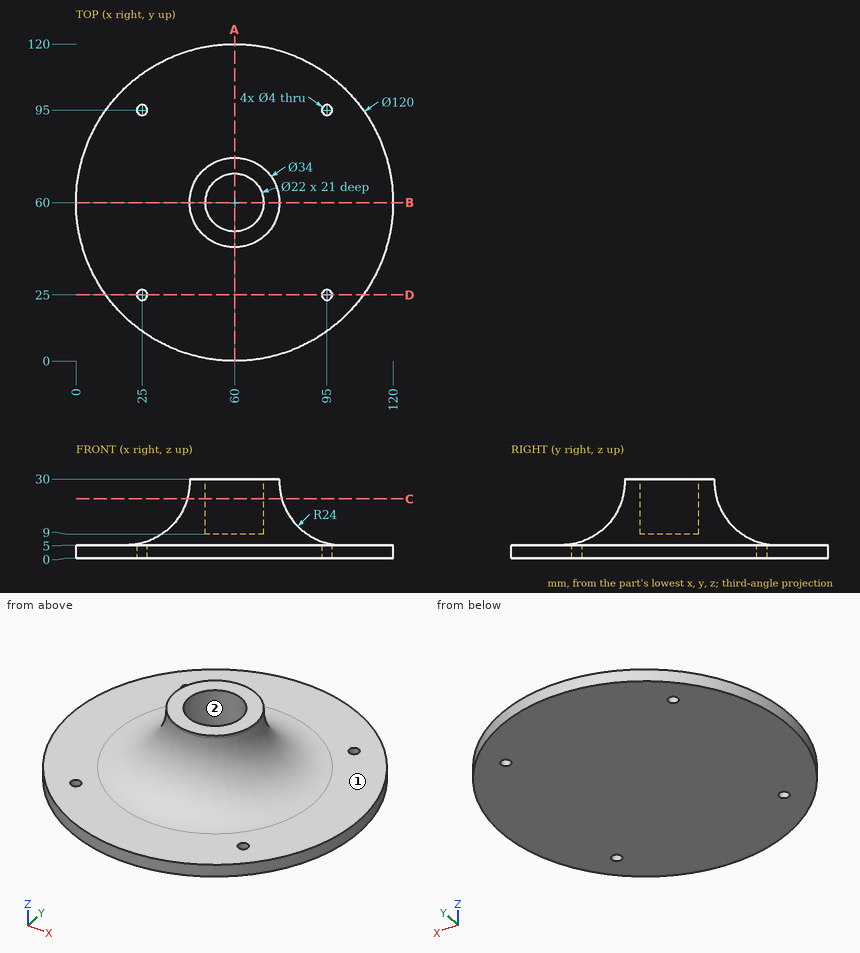
Source: three-view drawing plus pictorial views. Frame: mm from the lowest corner of the part. Round coordinates to 2 decimals unless told otherwise and drop trailing zeros. Loops run counter-clockwise (first coordinate to the right, second up) from the corner with the lowest first, then second, coordinate; pieces in that order, holes last.
1. Section query A-A on x = 60. Output: boundary loops of the cut face in (y, z).
2. Section query C-C on z = 22.5. Output: boundary loops of the cut face in (x, y).
3. Contact query for flat-ended pins moving along their axis: pin 1 (2.5 mm diameter, centred on x = 25, y = 95, fed in from -Z); pin 2 (6 mm diameter, centred on x = 76, y = 107, fed in from +Z); pin 3 (1.5 mm diameter, centred on y = 29.5, z = 5.5, fed in from -X); pin 4 (1 mm diameter, centred on x = 52, z = 11, fed in from -Y). Output: stop coordinate, or through.
4. Mould query, pull axis Y, two halves, no side actions, for the marked faces 1 and 2. Classes: released by +Y, released by -Y, zero draft, split by the parting line, or undercut.
5. Section query D-D on y = 25. Give the number of separate pieces and of enclosed holes in the cut face, and give its area (3 significant figures).
6. Ray query, L1, parallel to Y at x = 25, z = 3.1; L2, parallel to Z at x = 16.5, y = 29. Return the intervals inside material, ascending.
Answers below:
1. outline: (0, 0) - (120, 0) - (120, 5) - (101, 5) arc R24 cw to (77, 29) - (77, 30) - (71, 30) - (71, 9) - (49, 9) - (49, 30) - (43, 30) - (43, 29) arc R24 cw to (19, 5) - (0, 5) - close
2. outline: circle Ø35.79 at (60, 60); hole circle Ø22 at (60, 60)
3. pin 1: passes through
3. pin 2: stops at z = 5
3. pin 3: stops at x = 8
3. pin 4: stops at y = 35.54
4. face 1: zero draft
4. face 2: undercut
5. separate pieces: 3
5. enclosed holes: 0
5. area: 464 mm2
6. L1: y = 11.27 to 23, 27 to 93, 97 to 108.73
6. L2: z = 0 to 5
